For this review, take the finished solid that the model builds, in its own axes (mm). Face numbers are marked on the shaded views. A direction names the side the tool comes from. Give positions to 0.01 mm unless a question says otherwise; leave off trailing zeros. Loops run counter-clockwise (first coordinate to the right, second up) from the corner with the lowest first, then second, coordinate; pieces in that order, holes last. Notation, with made-up numbers: (-34.5, 30) - (0.5, 30) arc R17 ccw to (0.5, 51) - close; hole circle Ø3 at (69, -34). An arc over 180 degrees is marked (long way). Put each result on its own line as item: value.
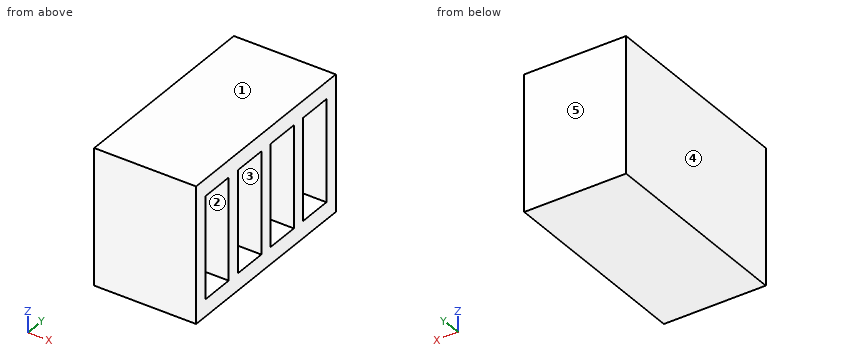
from build123d import *

# Parameters (mm, degrees)
F0_W     = 76.2
F0_H     = 152.4
F1_DEPTH = 101.6
F2_W     = 25.4
F2_H     = 76.2
F3_DEPTH = 50.8


with BuildPart() as f1:
    # F0 (on Top) → F1 (new body)
    with BuildSketch(Plane.XY):
        with Locations((0.829596, 34.125201)):
            Rectangle(F0_W, F0_H)
    extrude(amount=F1_DEPTH)

    # F2 (on face) → F3 (cut)
    with BuildSketch(Plane.YZ.offset(38.929596)):
        with Locations((87.465201, 50.8)):
            Rectangle(F2_W, F2_H)
        with Locations((51.905201, 50.8)):
            Rectangle(F2_W, F2_H)
        with Locations((16.345201, 50.8)):
            Rectangle(F2_W, F2_H)
        with Locations((-19.214799, 50.8)):
            Rectangle(F2_W, F2_H)
    extrude(amount=-F3_DEPTH, mode=Mode.SUBTRACT)


solid = f1.part
1) Take a section at A-A on x = 19.5. State the section outline as (y, z) points.
Geometry check:
outline: (-42.07, 0) - (110.33, 0) - (110.33, 101.6) - (-42.07, 101.6) - close; hole (-31.91, 12.7) - (-6.51, 12.7) - (-6.51, 88.9) - (-31.91, 88.9) - close; hole (3.65, 12.7) - (29.05, 12.7) - (29.05, 88.9) - (3.65, 88.9) - close; hole (39.21, 12.7) - (64.61, 12.7) - (64.61, 88.9) - (39.21, 88.9) - close; hole (74.77, 12.7) - (100.17, 12.7) - (100.17, 88.9) - (74.77, 88.9) - close
2) Wall thickness on line 1 (Y direction, x = -5.5, z = 68); line 2 (Z direction, x = 35.5, y = 94); line 3 (X direction, y = 45, z = 61.5): over which ranges is each line inside the solid? List them lowest first.
Geometry check:
line 1: y = -42.07 to -31.91, -6.51 to 3.65, 29.05 to 39.21, 64.61 to 74.77, 100.17 to 110.33
line 2: z = 0 to 12.7, 88.9 to 101.6
line 3: x = -37.27 to -11.87
3) Take a section at C-C on z = 16. State the section outline as (x, y) points, and give its area (3 significant figures).
Geometry check:
outline: (-37.27, -42.07) - (38.93, -42.07) - (38.93, -31.91) - (-11.87, -31.91) - (-11.87, -6.51) - (38.93, -6.51) - (38.93, 3.65) - (-11.87, 3.65) - (-11.87, 29.05) - (38.93, 29.05) - (38.93, 39.21) - (-11.87, 39.21) - (-11.87, 64.61) - (38.93, 64.61) - (38.93, 74.77) - (-11.87, 74.77) - (-11.87, 100.17) - (38.93, 100.17) - (38.93, 110.33) - (-37.27, 110.33) - close
area: 6,450 mm²
4) Take a section at B-B on y = -13.5. State the section outline as (x, z) points, and give its area (3 significant figures).
Geometry check:
outline: (-37.27, 0) - (38.93, 0) - (38.93, 12.7) - (-11.87, 12.7) - (-11.87, 88.9) - (38.93, 88.9) - (38.93, 101.6) - (-37.27, 101.6) - close
area: 3,870 mm²
5) For the marked faces 1 and 2, list the 3-axis set-ups (+Z, -Z, +X, -X, +Y, -Y) from which the entire face can be reached by the end or side of a thin tool; tool diameter is ignored.
Geometry check:
face 1: +Z, +X, -X, +Y, -Y
face 2: +X
6) Insertion check: pin 1 Ø12.5 at (y, z) = (18.5, 45) entering from +X. The pin has a flat end and moves straight along its axis. Give the tip position at first contact, or say it passes through.
Geometry check:
pin 1: stops at x = -11.87
7) Draft analysis for pull direction Y (two halves, no side actions). For the marked faces 3, 4 and 5, state which applies: pulls with the +Y half, pulls with the -Y half, needs draft (parallel to the pull), parting line crosses it, or undercut.
Geometry check:
face 3: undercut
face 4: needs draft
face 5: pulls with the +Y half
